For this review, take the finished solid that the model builds, in its own axes (mm). Give positions to 0.01 mm unless a question says otherwise; leave off trailing zeros. Order: outer loops, then holes, each group sorted by start corner. A loop starts at its lowest first (then second) coordinate and runs counter-clockwise, first axis right, second up.
Autodesk Inventor part; units mm, degrees
ref_plane "YZ Plane" through (0, 0, 0) normal (1, 0, 0) x (0, 1, 0)
ref_plane "XZ Plane" through (0, 0, 0) normal (0, 1, 0) x (-1, 0, 0)
ref_plane "XY Plane" through (0, 0, 0) normal (0, 0, 1) x (1, 0, 0)
sketch "Esquisse1" plane through (0, 0, 0) normal (0, 0, 1) x (1, 0, 0)
  arc A0 (22, 0) -> (10, 19.5959) centre (0, 0) ccw
  arc A1 (23, 0) -> (13, 18.9737) centre (0, 0) ccw
  line L0 (13, 18.9737) -> (13, 28.9737)
  line L1 (13, 28.9737) -> (10, 28.9737)
  line L2 (10, 28.9737) -> (10, 19.5959)
  line L3 (23, 0) -> (22, 0)
  dimension "d0" = 1
  dimension "d1" = 22
  dimension "d2" = 10
  dimension "d3" = 3
  dimension "d4" = 10
extrude "Extrusion1" add sketch "Esquisse1" along normal blind 8
sketch "Esquisse2" plane through (13, 18.9737, 0) normal (1, 0, 0) x (0, 0, -1)
  line L0 (0, 0) -> (0, 10)
  line L1 (0, 10) -> (-8, 10)
  line L2 (-8, 0) -> (-8, 10)
  line L3 (0, 0) -> (-8, 0)
  point P0 (0, -18.9737)
  point P1 (-4, 5)
  point P2 (0, 5)
  point P3 (-4, 10)
hole "Perçage1" at (13, 23.9737, 4) direction (-1, 0, 0) diameter 3.4 depth 3 counterbore diameter 6.5 counterbore depth 1
chamfer "Chanfrein1" distance 1 angle 45 4 edges at (13, 28.9737, 4) (11.5, 28.9737, 8) (11.5, 28.9737, 0) (13, 18.9737, 4)
mirror "Symétrie1" about plane through (22, 0, 0) normal (0, -1, 0) of "Extrusion1", "Perçage1", "Chanfrein1"
properties part number "guide_attache"
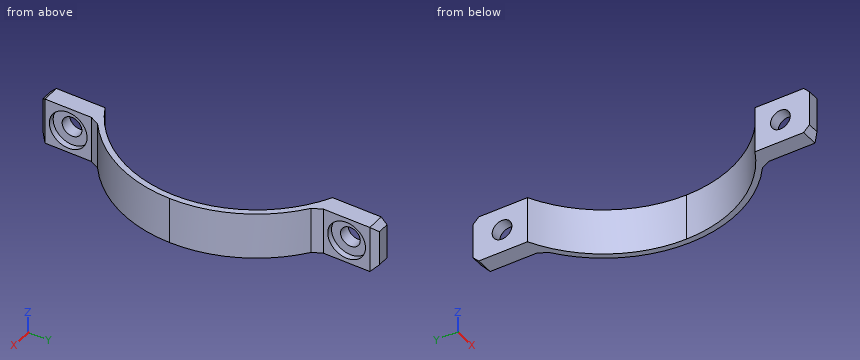
1) We need section C-C on x = 21.25. Give the boundary of the cut face in (y, z).
Answer sheet:
outline: (-8.8, 0) - (-5.7, 0) - (-5.7, 8) - (-8.8, 8) - close; (5.7, 0) - (8.8, 0) - (8.8, 8) - (5.7, 8) - close
2) Clearance check with flat-ended pins moving along their axes: pin 1 (1 mm diameter, centred on y = -1, z = 6, fed in from +X); pin 2 (4 mm diameter, centred on y = -23.97, z = 4, fed in from +X); pin 3 (4 mm diameter, centred on x = 19.5, y = -13.5, fed in from -Z); pin 4 (2.5 mm diameter, centred on y = -22.5, z = 2, fed in from +X). State where each tip first meets the part, or that it passes through.
Answer sheet:
pin 1: stops at x = 22.99
pin 2: stops at x = 12
pin 3: stops at z = 0
pin 4: stops at x = 13
3) We need section A-A on z = 4. Count the separate pieces of the cut face and the enclosed holes in it, then the cut area to 3 significant figures.
Answer sheet:
separate pieces: 3
enclosed holes: 0
area: 77.6 mm2
4) We need section B-B on x = 18. Give the boundary of the cut face in (y, z), then the cut area to 3 significant figures.
Answer sheet:
outline: (-14.32, 0) - (-12.65, 0) - (-12.65, 8) - (-14.32, 8) - close; (12.65, 0) - (14.32, 0) - (14.32, 8) - (12.65, 8) - close
area: 26.7 mm2
5) We need section D-D on z = 6.25. Give the boundary of the cut face in (x, y).
Answer sheet:
outline: (10, -28.97) - (12, -28.97) - (13, -27.97) - (13, -26.32) - (12, -26.32) - (12, -21.63) - (13, -21.63) - (13, -19.97) - (13.81, -18.39) arc R23 ccw to (23, 0) arc R23 ccw to (13.81, 18.39) - (13, 19.97) - (13, 21.63) - (12, 21.63) - (12, 26.32) - (13, 26.32) - (13, 27.97) - (12, 28.97) - (10, 28.97) - (10, 19.6) arc R22 cw to (22, 0) arc R22 cw to (10, -19.6) - close
6) To check wall thickness, follow line 1 (Y direction, x = 12.35, z = 4); line 2 (Y direction, x = 12.65, z = 4); line 3 (Y direction, x = 13.5, z = 2.5). State the ranges of each line that lie inside material, in increasing order.
Answer sheet:
line 1: y = -28.62 to -27.22, -20.72 to -18.21, 18.21 to 20.72, 27.22 to 28.62
line 2: y = -28.32 to -27.22, -20.72 to -18, 18 to 20.72, 27.22 to 28.32
line 3: y = -19 to -17.37, 17.37 to 19
